Design review of the part built by this model. Coordinates are the model's own, in mm. A direction names the side the tool comes from. Give positions to 0.01 mm unless a question says otherwise; leave off trailing zeros. Write each loop counter-clockwise with the first axis right and the second up, starting at its lowest first coordinate (ties: lowest second). Pieces come first, ordered by that corner, then holes. Notation, with made-up numbers: M 64.25,-28.75 L 119.25,-28.75 A23 ccw 119.25,-18.75 Z; hole C 79,-31.5 d3. An arc over 180 degrees is marked long. Answer in a Markdown table with one row per item.
Autodesk Inventor part; units mm, degrees
ref_plane "Płaszczyzna konstrukcyjna1" through (-12.2191, -12.0493, 11.96) normal (0, 0, -1) x (-0.4239, 0.9057, 0)
ref_plane "Płaszczyzna konstrukcyjna2" through (-9.0993, -8.9295, 0) normal (0, 0, 1) x (1, 0, 0)
ref_plane "YZ Plane" through (0, 0, 0) normal (1, 0, 0) x (0, 1, 0)
sketch "Szkic1" plane through (0, 0, 0) normal (0, 0, 1) x (1, 0, 0)
  circle A0 centre (-2.912, -2.7423) radius 5.3
  circle A1 centre (-2.912, -2.7423) radius 5
  point P0 (0, 0)
  dimension "d0" = 10
extrude "Wyciągnięcie proste1" add sketch "Szkic1" along normal blind 120 contours A1
sketch "Szkic2" plane through (-2.912, -2.7423, 5) normal (0, 0, -1) x (-1, 0, 0)
  circle A0 centre (0, 0) radius 5
  circle A1 centre (0, 0) radius 4.284
  point P0 (-2.912, 2.7423)
ref_plane "Płaszczyzna konstrukcyjna1" through (-12.2191, -12.0493, 11.96) normal (0, 0, -1) x (-0.4239, 0.9057, 0)
extrude "Wyciągnięcie proste2" cut sketch "Szkic2" against normal up to surface (6.96 mm away)
extrude "Wyciągnięcie proste3" cut sketch "Szkic2" against normal blind 5 contours A1
sketch "Szkic3" plane through (-2.912, -2.7423, 10) normal (0, 0, -1) x (-1, 0, 0)
  circle A0 centre (0, 0) radius 4.284
  circle A1 centre (0, 0) radius 4.284
  circle A2 centre (0, 0) radius 5
  point P0 (-2.912, 2.7423)
ref_plane "Płaszczyzna konstrukcyjna2" through (-9.0993, -8.9295, 0) normal (0, 0, 1) x (1, 0, 0)
extrude "Wyciągnięcie proste4" add sketch "Szkic3" along normal up to surface (10 mm away) contours A0 | A2
sketch "Szkic4" plane through (-2.912, -2.7423, 11.96) normal (0, 0, -1) x (-1, 0, 0)
  circle A0 centre (0, 0) radius 5
  circle A1 centre (0, 0) radius 6
  point P0 (-2.912, 2.7423)
  dimension "d15" = 12
extrude "Wyciągnięcie proste5" add sketch "Szkic4" along normal blind 2 contours A0 | A1
sketch "Szkic5" plane through (-2.912, -2.7423, 9.96) normal (0, 0, -1) x (-1, 0, 0)
  circle A0 centre (0, 0) radius 5
  circle A1 centre (0, 0) radius 5
  circle A2 centre (0, 0) radius 5
  point P0 (-2.912, 2.7423)
extrude "Wyciągnięcie proste6" add sketch "Szkic5" along normal blind 25
sketch "Szkic6" plane through (-2.912, -2.7423, 116) normal (0, 0, 1) x (1, 0, 0)
  circle A0 centre (0, 0) radius 5
  point P0 (2.912, 2.7423)
extrude "Wyciągnięcie proste7" add sketch "Szkic6" along normal blind 15
sketch "Szkic7" plane through (-2.912, -2.7423, 131) normal (0, 0, 1) x (1, 0, 0)
  circle A0 centre (0, 0) radius 5
  point P0 (2.912, 2.7423)
extrude "Wyciągnięcie proste8" cut sketch "Szkic7" against normal blind 0.04
properties part number "wał_2"
1) For faces 1 (the face through (1, 1, 11.96)), 2 (the face through (-2.13, -8.69, 10.97)), 3 (the face through (1, 1, 9.96)), list the 3-axis set-ups (+Z, -Z, +X, -X, +Y, -Y) from which the entire face can be reached by the end or side of a thin tool; tool diameter is ignored.
Geometry says:
| item | result |
|---|---|
| face 1 | +Z |
| face 2 | +Z, -Z |
| face 3 | -Z |
2) Add section B-B (x = -2.25). Write out the cut boundary in (y, z).
Geometry says:
| item | result |
|---|---|
| outline | M -8.71,9.96 L -7.7,9.96 L -7.7,-15.04 L 2.21,-15.04 L 2.21,9.96 L 3.22,9.96 L 3.22,11.96 L 2.21,11.96 L 2.21,130.96 L -7.7,130.96 L -7.7,11.96 L -8.71,11.96 Z |
3) To check wall thickness, follow probe 1 along X at (y, z) = (-3, 87.5); probe 2 along Z at (x, y) = (2.25, -0.5); probe 3 along Y at (x, z) = (-2.75, 22.5). State the ranges of each line that lie inside material, in increasing order. Write a range as [from, to].
Geometry says:
| item | result |
|---|---|
| probe 1 | [-7.91, 2.08] |
| probe 2 | [9.96, 11.96] |
| probe 3 | [-7.74, 2.26] |
4) Insertion check: P1, Ø6, axis at y = -2.5, z = 70, coming from the -X side; P2, Ø5, axis at x = -1.5, z = 110.5, coming from the +Y side; P3, Ø6, axis at y = -7.5, z = 27, coming from the -X side. Each pin has a flat end and moves straight along its axis. Give the tip position at first contact, or say it passes through.
Geometry says:
| item | result |
|---|---|
| P1 | x = -7.91 |
| P2 | y = 2.26 |
| P3 | x = -7.59 |
5) Add section A-A (y = -1.5). Write out the cut boundary in (x, z).
Geometry says:
| item | result |
|---|---|
| outline | M -8.78,9.96 L -7.76,9.96 L -7.76,-15.04 L 1.93,-15.04 L 1.93,9.96 L 2.96,9.96 L 2.96,11.96 L 1.93,11.96 L 1.93,130.96 L -7.76,130.96 L -7.76,11.96 L -8.78,11.96 Z |
6) Add section C-C (z = 103). Write out the cut boundary in (x, y).
Geometry says:
| item | result |
|---|---|
| outline | C -2.91,-2.74 d10 |
